Part model, mm, in its own coordinate system. Coordinates: 2 decimals unless noted, no trailing zeros. Loops run counter-clockwise (first coordinate to the right, second up) from the corner with the lowest first, then second, coordinate; pieces in that order, holes last. Notation, with made-up numbers: (-32, 11) - (-16, 11) arc R20 cw to (-16, 36) - close; hole circle Ø3 at (77, 44.25). An arc over 180 degrees is marked (long way). Answer as CSV lines item,"result".
from build123d import *

# Parameters (mm, degrees)
SKETCH008_R   = 54
SKETCH008_R_2 = 40
PAD005_DEPTH  = 25
FILLET_R      = 3
CHAMFER_SIZE  = 1


with BuildPart() as part:
    # Sketch008 → Pad005 (new body, symmetric)
    with BuildSketch(Plane.YZ):
        Circle(SKETCH008_R)
        Circle(SKETCH008_R_2, mode=Mode.SUBTRACT)
    extrude(amount=PAD005_DEPTH, both=True)

    # Fillet
    fillet_edges = [part.edges().sort_by_distance(p)[0] for p in [
        (-25, -54, 0),
        (25, -54, 0),
    ]]
    fillet(fillet_edges, radius=FILLET_R)

    # Chamfer
    chamfer_edges = [part.edges().sort_by_distance(p)[0] for p in [
        (-25, -40, 0),
        (0, 40, 0),
        (25, -40, 0),
    ]]
    chamfer(chamfer_edges, length=CHAMFER_SIZE)


solid = part.part
Q1. Saw through at A-A (y = 0). Give the cut face in (x, z), then the cut area to 3 significant figures.
Results:
outline,"(-25, -51) arc R3 ccw to (-22, -54) - (22, -54) arc R3 ccw to (25, -51) - (25, -41) - (24, -40) - (-24, -40) - (-25, -41) - close; (-25, 41) - (-24, 40) - (24, 40) - (25, 41) - (25, 51) arc R3 ccw to (22, 54) - (-22, 54) arc R3 ccw to (-25, 51) - close"
area,"1,390 mm^2"
Q2. Wall check: L1, parallel to Z at x = 8, y = 0; L2, parallel to Y at x = -4, z = 1; L3, parallel to Z at x = -8.5, y = 24. Give the ranges that are in metal, low to high.
Results:
L1,"z = -54 to -40, 40 to 54"
L2,"y = -53.99 to -39.99, 39.99 to 53.99"
L3,"z = -48.37 to -32, 32 to 48.37"
Q3. Two-plate mould, pull along Y, no slides. Class faces 1 (the face through (-0.34, -8.67, -39.05)), 2 (the face through (25, -34.2, 22.9)), 3 (the face through (0.308, -11.706, -52.716)): released by +Y, released by -Y, zero draft, split by the parting line, or undercut.
Results:
face 1,"undercut"
face 2,"zero draft"
face 3,"split by the parting line"
Q4. Flat gauge pins, fed straight in: pin 1 (1 mm diameter, centred on x = -4.5, y = 18, fed in from +Z); pin 2 (1.5 mm diameter, centred on x = 3, y = -10, fed in from +Z); pin 3 (1 mm diameter, centred on x = -4, y = -12, fed in from +Z). Where does each tip first touch, or does it go through?
Results:
pin 1,"stops at z = 51.09"
pin 2,"stops at z = 53.2"
pin 3,"stops at z = 52.76"
Q5. Saw through at C-C (x = -6). Give the cut face in (y, z).
Results:
outline,"circle Ø108 at (0, 0); hole circle Ø80 at (0, 0)"
